```python
from build123d import *

# Parameters (mm, degrees)
BOSS_EXTRUDE1_DEPTH = 3.175


with BuildPart() as part:
    # Sketch1 → Boss-Extrude1 (new body)
    with BuildSketch(Plane.XY):
        Polygon((3.175, 27.5), (0, 27.5), (0, 38), (3.175, 38), (3.175, 42), (0, 42), (0, 52.5), (3.175, 52.5), (3.175, 58.4125), (36.7, 58.4125), (36.7, 52.5), (39.875, 52.5), (39.875, 42), (36.7, 42), (36.7, 38), (39.875, 38), (39.875, 27.5), (36.7, 27.5), (36.7, 21.5875), (3.175, 21.5875), align=None)
        Polygon((32.7, 40), (7.175, 50.110154656), (7.175, 29.889845344), align=None, mode=Mode.SUBTRACT)
        Polygon((32.7, 54.4125), (7.175, 54.4125), (32.7, 44.302345344), align=None, mode=Mode.SUBTRACT)
        Polygon((32.7, 25.5875), (32.7, 35.697654656), (7.175, 25.5875), align=None, mode=Mode.SUBTRACT)
    extrude(amount=BOSS_EXTRUDE1_DEPTH)


solid = part.part
```
Model file for the job. Use its own axes, mm. A direction names the side the tool comes from. Coordinates: 2 decimals unless noted, no trailing zeros. Order: outer loops, then holes, each group sorted by start corner. A loop starts at its lowest first (then second) coordinate and runs counter-clockwise, first axis right, second up. Notation, with made-up numbers: (84, -33) -> (119, -33) arc R28 ccw to (119, -9) -> close; hole circle Ø9 at (73, -38). An arc over 180 degrees is marked (long way). Return JSON: item names as keys, results as strings.
Item 1: 3-axis set-ups, long thin cutter, end or side, ignore diameter. For faces 1 (the face through (36.7, 25, 2)), 2 (the face through (19.759, 49.428, 1.565)), 3 (the face through (2, 27.5, 2)), 4 (the face through (38, 38, 2)): which of +Z, -Z, +X, -X, +Y, -Y reach the whole face in a straight line?
Model answer:
{"face 1": "+Z, -Z, +X, -Y", "face 2": "+Z, -Z", "face 3": "+Z, -Z, -X, -Y", "face 4": "+Z, -Z, +X"}
Item 2: Wall check: line 1 along Y through (x, z) = (25, 0.8); line 2 along Y through (x, z) = (23.5, 2.75); line 3 along Y through (x, z) = (2.5, 0.9). Give the ranges that are in metal, low to high. Write a range as from..to.
Model answer:
{"line 1": "y = 21.59..25.59, 32.65..36.95, 43.05..47.35, 54.41..58.41", "line 2": "y = 21.59..25.59, 32.05..36.36, 43.64..47.95, 54.41..58.41", "line 3": "y = 27.5..38, 42..52.5"}
Item 3: Pin check, flat tips, straight feed: P1, Ø1, axis at x = 2, z = 1, coming from the +Y side; P2, Ø1.6, axis at y = 40.5, z = 2, coming from the -X side (3 decimals); P3, Ø1, axis at y = 55.5, z = 1.5, coming from the +X side. Stop position of each tip, or through.
Model answer:
{"P1": "stops at y = 52.5", "P2": "stops at x = 3.175", "P3": "stops at x = 36.7"}
Item 4: Slice it at B-B (x = 21). Write the cut outline in (y, z) (1 decimal), then the cut area to 3 significant figures.
Model answer:
{"outline": "(21.6, 0) -> (25.6, 0) -> (25.6, 3.2) -> (21.6, 3.2) -> close; (31.1, 0) -> (35.4, 0) -> (35.4, 3.2) -> (31.1, 3.2) -> close; (44.6, 0) -> (48.9, 0) -> (48.9, 3.2) -> (44.6, 3.2) -> close; (54.4, 0) -> (58.4, 0) -> (58.4, 3.2) -> (54.4, 3.2) -> close", "area": "52.7 mm²"}
Item 5: Slice it at A-A (z = 1.2). Count the separate pieces of the cut face and the enclosed holes in it, then the cut area to 3 significant figures.
Model answer:
{"separate pieces": "1", "enclosed holes": "3", "area": "852 mm²"}
Item 6: Slice it at D-D (y = 32). Write the cut outline in (x, z) (3 decimals), then the cut area to 3 significant figures.
Model answer:
{"outline": "(0, 0) -> (7.175, 0) -> (7.175, 3.175) -> (0, 3.175) -> close; (12.502, 0) -> (23.365, 0) -> (23.365, 3.175) -> (12.502, 3.175) -> close; (32.7, 0) -> (39.875, 0) -> (39.875, 3.175) -> (32.7, 3.175) -> close", "area": "80.0 mm²"}
Item 7: Mould opens along Y. For faces 5 (the face through (38, 52.5, 2)), 6 (the face through (3.175, 40, 2)), 7 (the face through (3.175, 25, 2)) say: pulls with the +Y half, pulls with the -Y half, needs draft (parallel to the pull), parting line crosses it, or undercut.
Model answer:
{"face 5": "pulls with the +Y half", "face 6": "undercut", "face 7": "needs draft"}
Item 8: Slice it at C-C (y = 41.5). Write the cut outline in (x, z) (3 decimals), then the cut area to 3 significant figures.
Model answer:
{"outline": "(3.175, 0) -> (7.175, 0) -> (7.175, 3.175) -> (3.175, 3.175) -> close; (28.913, 0) -> (36.7, 0) -> (36.7, 3.175) -> (28.913, 3.175) -> close", "area": "37.4 mm²"}
